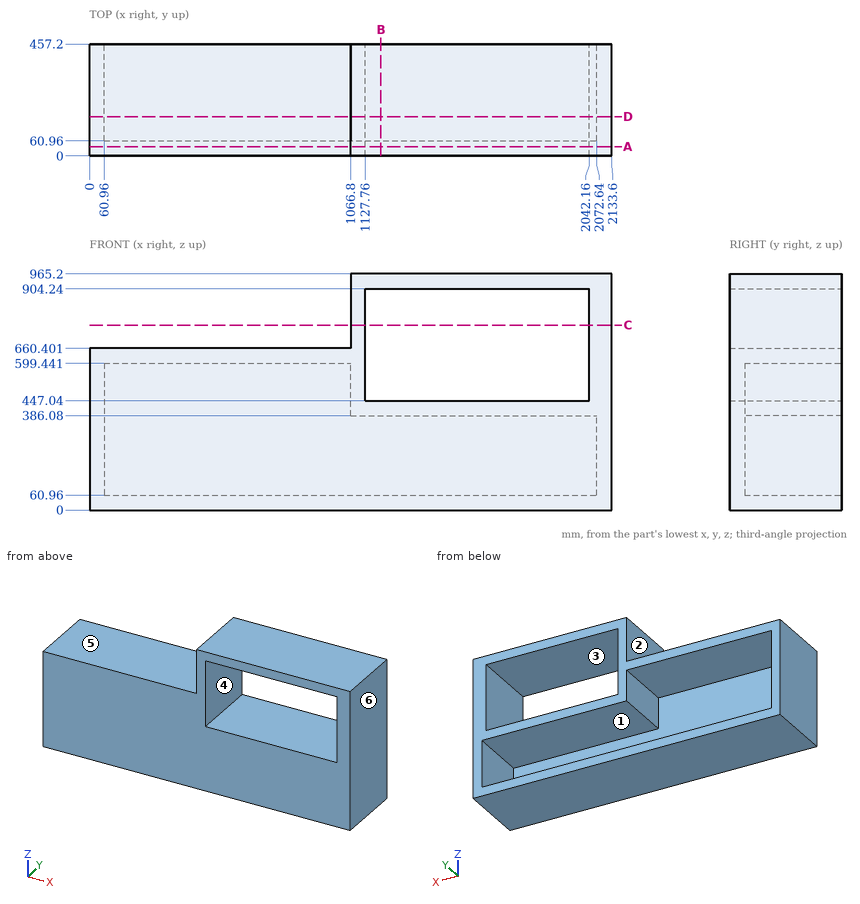
Drawing for the job (mm, zero at the part's lowest x, y, z). A direction names the side the tool comes from. Round coordinates to 2 decimals unless told otherwise and drop trailing zeros. Loops run counter-clockwise (first coordinate to the right, second up) from the corner with the lowest first, then second, coordinate; pieces in that order, holes last. Notation, with made-up numbers: (56.25, 49) -> (106.25, 49) arc R34 cw to (106.25, 84) -> close; hole circle Ø10 at (67.25, 78). An arc over 180 degrees is marked (long way). Answer as CSV lines item,"result". Start each with the question number.
1) Probe line 1 along Z through (x, y) = (1516, 310); line 2 along X through (y, z) = (101.5, 466.5); line 3 along Z through (x, y) = (700.5, 388.5). List the from-to ranges inside material, lowest first.
2) Tool access for the marked faces 1, 2 and 3: list every direction of +Z, -Z, +X, -X, +Y, -Y with a clear straight run to the whole face (end or side of a thin tool).
3) Slice it at D-D (y = 160). List the corners of the cut face in (x, z), plus the area to 3 significant figures.
4) Slice it at C-C (z = 756). List the corners of the cut face in (x, y).
5) Slice it at A-A (y = 37.5). List the corners of the cut face in (x, z).
6) Mould opens along Z. For the marked faces 4, 5 and 6 say: +Z half, -Z half, draft (parallel to the pull), parting line (faces both ways), or undercut.
7) Slice it at B-B (x = 1190.5). List the corners of the cut face in (y, z), plus the area to 3 significant figures.
8) Pin check, flat tips, straight feed: P1, Ø4, axis at y = 110, z = 735, coming from the -X side; P2, Ø10, axis at x = 1398, z = 230, coming from the +Y side. Stop position of each tip, or through.
Filled in:
1,line 1,"z = 0 to 60.96, 386.08 to 447.04, 904.24 to 965.2"
1,line 2,"x = 0 to 60.96, 1066.8 to 1127.76, 2042.16 to 2133.6"
1,line 3,"z = 0 to 60.96, 599.44 to 660.4"
2,face 1,"+Y"
2,face 2,"+Z, -X, +Y, -Y"
2,face 3,"+Y, -Y"
3,outline,"(0, 0) -> (2133.6, 0) -> (2133.6, 965.2) -> (1066.8, 965.2) -> (1066.8, 660.4) -> (0, 660.4) -> close; hole (60.96, 60.96) -> (2072.64, 60.96) -> (2072.64, 386.08) -> (1066.8, 386.08) -> (1066.8, 599.44) -> (60.96, 599.44) -> close; hole (1127.76, 447.04) -> (2042.16, 447.04) -> (2042.16, 904.24) -> (1127.76, 904.24) -> close"
3,area,"447,000 mm2"
4,outline,"(1066.8, 0) -> (1127.76, 0) -> (1127.76, 457.2) -> (1066.8, 457.2) -> close; (2042.16, 0) -> (2133.6, 0) -> (2133.6, 457.2) -> (2042.16, 457.2) -> close"
5,outline,"(0, 0) -> (2133.6, 0) -> (2133.6, 965.2) -> (1066.8, 965.2) -> (1066.8, 660.4) -> (0, 660.4) -> close; hole (1127.76, 447.04) -> (2042.16, 447.04) -> (2042.16, 904.24) -> (1127.76, 904.24) -> close"
6,face 4,"undercut"
6,face 5,"+Z half"
6,face 6,"draft"
7,outline,"(0, 0) -> (457.2, 0) -> (457.2, 60.96) -> (60.96, 60.96) -> (60.96, 386.08) -> (457.2, 386.08) -> (457.2, 447.04) -> (0, 447.04) -> close; (0, 904.24) -> (457.2, 904.24) -> (457.2, 965.2) -> (0, 965.2) -> close"
7,area,"103,000 mm2"
8,P1,"stops at x = 1066.8"
8,P2,"stops at y = 60.96"
